from build123d import *

# Parameters (mm, degrees)
F0_R     = 11.125
F1_DEPTH = 7


with BuildPart() as f1:
    # F0 (on Top) → F1 (new body)
    with BuildSketch(Plane.XY):
        with BuildLine():
            ThreePointArc((2.037572, -33.564942), (8.556682, -29.737896), (11.125, -22.628127))
            ThreePointArc((11.125, -22.628127), (10.55403, -19.109877), (8.899727, -15.952762))
            ThreePointArc((8.899727, -15.952762), (-1.46999, -11.600672), (-10.337576, -18.517148))
            ThreePointArc((-10.337576, -18.517148), (-10.522788, -19.112066), (-10.732419, -19.698825))
            ThreePointArc((-10.732419, -19.698825), (-9.425257, -28.538301), (-2.037572, -33.564942))
            ThreePointArc((-2.037572, -33.564942), (0, -33.626731), (2.037572, -33.564942))
        make_face()
        with BuildLine():
            ThreePointArc((-10.337576, -18.517148), (-1.46999, -11.600672), (8.899727, -15.952762))
            ThreePointArc((8.899727, -15.952762), (12.080882, -5.568253), (21.215107, 0.307436))
            ThreePointArc((21.215107, 0.307436), (10.78902, 4.517495), (9.359899, 15.670319))
            ThreePointArc((9.359899, 15.670319), (0.096944, 12.613685), (-9.250085, 15.402663))
            ThreePointArc((-9.250085, 15.402663), (-8.667904, 13.395096), (-8.471533, 11.314063))
            ThreePointArc((-8.471533, 11.314063), (-12.324704, 2.894673), (-21.215107, 0.307436))
            ThreePointArc((-21.215107, 0.307436), (-11.768489, -6.788973), (-10.337576, -18.517148))
        make_face()
        Circle(F0_R, mode=Mode.SUBTRACT)
        with BuildLine():
            ThreePointArc((-2.037572, -33.564942), (0, -33.753127), (2.037572, -33.564942))
            ThreePointArc((2.037572, -33.564942), (0, -33.626731), (-2.037572, -33.564942))
        make_face()
        with BuildLine():
            ThreePointArc((-10.732419, -19.698825), (-10.522788, -19.112066), (-10.337576, -18.517148))
            ThreePointArc((-10.337576, -18.517148), (-10.551553, -19.102455), (-10.732419, -19.698825))
        make_face()
        with BuildLine():
            ThreePointArc((9.359899, 15.670319), (10.78902, 4.517495), (21.215107, 0.307436))
            ThreePointArc((21.215107, 0.307436), (28.015923, 4.042235), (30.721533, 11.314063))
            ThreePointArc((30.721533, 11.314063), (30.561721, 13.192963), (30.086878, 15.017882))
            ThreePointArc((30.086878, 15.017882), (29.121603, 16.813365), (28.049307, 18.54706))
            ThreePointArc((28.049307, 18.54706), (17.904065, 22.30957), (9.359899, 15.670319))
        make_face()
        with BuildLine():
            ThreePointArc((-30.086878, 15.017882), (-29.123116, 5.568645), (-21.215107, 0.307436))
            ThreePointArc((-21.215107, 0.307436), (-12.324704, 2.894673), (-8.471533, 11.314063))
            ThreePointArc((-8.471533, 11.314063), (-8.667904, 13.395096), (-9.250085, 15.402663))
            ThreePointArc((-9.250085, 15.402663), (-17.761238, 22.286634), (-28.049307, 18.54706))
            ThreePointArc((-28.049307, 18.54706), (-29.121603, 16.813365), (-30.086878, 15.017882))
        make_face()
        with BuildLine():
            ThreePointArc((-28.049307, 18.54706), (-29.231065, 16.876563), (-30.086878, 15.017882))
            ThreePointArc((-30.086878, 15.017882), (-29.121603, 16.813365), (-28.049307, 18.54706))
        make_face()
        with BuildLine():
            ThreePointArc((30.086878, 15.017882), (29.231065, 16.876563), (28.049307, 18.54706))
            ThreePointArc((28.049307, 18.54706), (29.121603, 16.813365), (30.086878, 15.017882))
        make_face()
    extrude(amount=F1_DEPTH)


solid = f1.part
Verification items for the finished model (mm, model axes). Coordinates: 2 decimals unless noted, no trailing zeros. Loops run counter-clockwise (first coordinate to the right, second up) from the corner with the lowest first, then second, coordinate; pieces in that order, holes last. Notation, with made-up numbers: (75, 21.5) -> (103, 21.5) arc R14 ccw to (103, 34.5) -> close; hole circle Ø2 at (52.5, 66.5). An arc over 180 degrees is marked (long way). Answer as a JSON object with one key per item and string values. Group by question number.
Item 1: Sectioned sample at D-D on x = -24. Record the boundary of the cut face in (y, z).
Item 2: Sectioned sample at B-B on y = -4. Record the boundary of the cut face in (x, z).
Item 3: Scan lines: probe 1 along Y at (x, z) = (0, 1.75) (3 decimals); probe 2 along X at (y, z) = (-14, 3.25); probe 3 along X at (y, z) = (16.5, 3). Record each from-to range of solid material in increasing order.
Item 4: Mould release check, pull along Y, two halves, no side actions. Record for faces 1 (the cylindrical face through (27.943, 3.959, 3.451)), 2 (the cylindrical face through (18.061, 22.333, 3.451)), 3 (the cylindrical face through (11.99, -5.69, 3.45)), 4 (the cylindrical face through (-8.2, 7.52, 3.45)): +Y half, -Y half, draft (parallel to the pull), parting line (faces both ways), or undercut.
Item 5: Depth check by flat-ended pin: pin 1 (2 mm diameter, centred on x = -22.5, z = 5, fed in from -Y); pin 2 (2 mm diameter, centred on y = -27.5, z = 1.5, fed in from +X); pin 3 (4 mm diameter, centred on y = 15.5, z = 4.5, fed in from -X); pin 4 (13.5 mm diameter, centred on x = 0, y = 0, fed in from +Z). Enter the tip coordinate at first touch or a pass-through.
Item 6: Sectioned sample at C-C on x = -5. Record the boundary of the cut face in (y, z).
Evaluation:
{
 "1": {"outline": "(1.1, 0) -> (21.53, 0) -> (21.53, 7) -> (1.1, 7) -> close"},
 "2": {"outline": "(-13.84, 0) -> (-10.38, 0) -> (-10.38, 7) -> (-13.84, 7) -> close; (10.38, 0) -> (13.44, 0) -> (13.44, 7) -> (10.38, 7) -> close"},
 "3": {"probe 1": "y = -33.753 to -11.125, 11.125 to 12.613", "probe 2": "x = -9.75 to 8.92", "probe 3": "x = -29.44 to -9.75, 9.75 to 29.44"},
 "4": {"face 1": "-Y half", "face 2": "+Y half", "face 3": "undercut", "face 4": "undercut"},
 "5": {"pin 1": "stops at y = 0.35", "pin 2": "stops at x = 10.43", "pin 3": "stops at x = -30.5", "pin 4": "passes through"},
 "6": {"outline": "(-32.57, 0) -> (-9.94, 0) -> (-9.94, 7) -> (-32.57, 7) -> close; (9.94, 0) -> (13.36, 0) -> (13.36, 7) -> (9.94, 7) -> close"}
}
